Autodesk Inventor part; units mm, degrees
ref_plane "YZ Plane" through (0, 0, 0) normal (1, 0, 0) x (0, 1, 0)
ref_plane "XZ Plane" through (0, 0, 0) normal (0, 1, 0) x (-1, 0, 0)
ref_plane "XY Plane" through (0, 0, 0) normal (0, 0, 1) x (1, 0, 0)
sketch "Boceto1" plane through (0, 0, 0) normal (0, 0, 1) x (1, 0, 0)
  line L0 (0, 0) -> (-25.435, 0)
  line L1 (-25.435, 0) -> (-25.435, 10.53)
  line L2 (0, 0) -> (0, 11.4) construction
  arc A0 (9.5801, 10.53) -> (-9.5801, 10.53) centre (0, 16.38) ccw
  circle A1 centre (0, 16.38) radius 4.98
  line L3 (-25.435, 10.53) -> (-9.5801, 10.53)
  line L4 (0, 0) -> (25.435, 0)
  line L5 (25.435, 0) -> (25.435, 10.53)
  line L6 (25.435, 10.53) -> (9.5801, 10.53)
  dimension "d4" = 9.96
  dimension "d0" = 25.435
  dimension "d1" = 10.53
  dimension "d2" = 11.4
  dimension "d3" = 22.45
extrude "Extrusión1" add sketch "Boceto1" along normal blind 9.95
sketch "Boceto2" plane through (-25.435, 0, 0) normal (0, -1, 0) x (1, 0, 0)
  line L0 (25.435, 0) -> (25.435, 9.95) construction
  line L1 (36.66, 9.95) -> (14.21, 9.95)
  line L2 (25.435, 4.975) -> (41.935, 4.975) construction
  line L3 (41.935, 4.975) -> (43.685, 4.975) construction
  circle A0 centre (43.685, 4.975) radius 1.75
  circle A1 centre (7.185, 4.975) radius 1.75
  point P0 (35.0151, 9.95)
  point P1 (15.8549, 9.95)
  dimension "d7" = 16.5
  dimension "d8" = 1.75
extrude "Extrusión2" cut sketch "Boceto2" against normal up to surface (10.53 mm away)
properties part number "003" material "Steel"
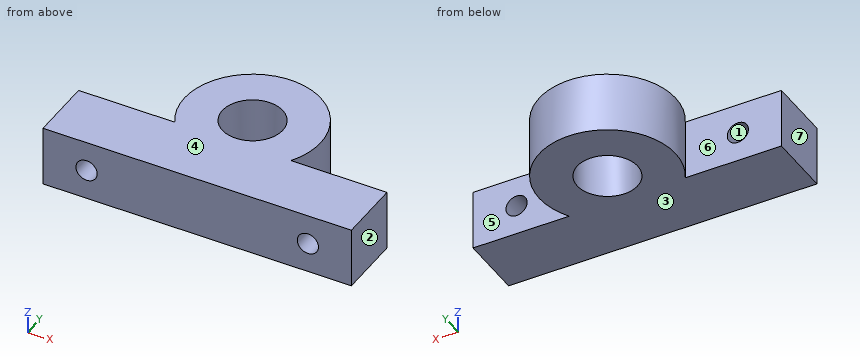
Can you work these out from the model? Positions are in its coordinate system, mm. Face numbers are marked on the shaded views. A direction names the side the tool comes from. Coordinates: 2 decimals unless noted, no trailing zeros. Loops run counter-clockwise (first coordinate to the right, second up) from the corner with the lowest first, then second, coordinate; pieces in that order, holes last. Notation, with made-up numbers: M 24,18.5 L 41,18.5 A29 cw 41,49.5 Z; hole C 40,-6 d11. An arc over 180 degrees is marked long. Return JSON: item names as keys, results as strings. Group by question number.
Item 1: On a 3-axis mill with a long thin cutter (end or side, diameter ignored), from which of +Z, -Z, +X, -X, +Y, -Y can I reach the whole of each face in a straight line? I mean the marked faces 5, 6 and 7. Say none if no direction works.
Item 2: Imagine slicing it at D-D (z = 4.25). Please give me the cut outline in (x, y) (3 decimals).
Item 3: I'm going to push flat-ended pins straight in: pin 1 Ø3 at (x, z) = (-16.5, 4.5) entering from -Y; pin 2 Ø3 at (x, z) = (-18.5, 5.5) entering from +Y. Where does each tip first touch, or does it pass through?
Item 4: Imagine slicing it at B-B (x = 0). Please give me the cut outline in (y, z) (3 decimals).
Item 5: Imagine slicing it at A-A (y = 16.38). Please give me the cut outline in (x, z) (3 decimals), and give its area (3 significant figures).
Item 6: Imagine slicing it at C-C (z = 8.75). Please give me the cut outline in (x, y) (3 decimals), and give its area (3 significant figures).
Item 7: Thinking about a two-plate mould opening in Z: for the marked faces 1, 2, 3 and 4, which applies, released by +Z, released by -Z, zero draft, split by the parting line, or undercut?
Item 8: If I drill on L1, parallel to Z at x = -18.25, y = 7.5 (3 decimals); L2, parallel to X at y = 6.75, z = 3.5 (3 decimals); L3, parallel to X at y = 2.5, z = 5.5 (3 decimals), over which ranges is the centre line in solid material (lowest first)? Write a range as from..to.
Verdict:
{
 "1": {"face 5": "+Z, -Z, +X", "face 6": "+Z, -Z, -X", "face 7": "+Z, -Z, -X, +Y, -Y"},
 "2": {"outline": "M -25.435,0 L -19.843,0 L -19.843,10.53 L -25.435,10.53 Z; M -16.657,0 L 16.657,0 L 16.657,10.53 L 9.58,10.53 A11.225 ccw long -9.58,10.53 L -16.657,10.53 Z; M 19.843,0 L 25.435,0 L 25.435,10.53 L 19.843,10.53 Z; hole C 0,16.38 d9.96"},
 "3": {"pin 1": "stops at y = 0", "pin 2": "stops at y = 10.53"},
 "4": {"outline": "M 0,0 L 11.4,0 L 11.4,9.95 L 0,9.95 Z; M 21.36,0 L 27.605,0 L 27.605,9.95 L 21.36,9.95 Z"},
 "5": {"outline": "M -11.225,0 L -4.98,0 L -4.98,9.95 L -11.225,9.95 Z; M 4.98,0 L 11.225,0 L 11.225,9.95 L 4.98,9.95 Z", "area": "124 mm^2"},
 "6": {"outline": "M -25.435,0 L 25.435,0 L 25.435,10.53 L 9.58,10.53 A11.225 ccw long -9.58,10.53 L -25.435,10.53 Z; hole C 0,16.38 d9.96", "area": "781 mm^2"},
 "7": {"face 1": "undercut", "face 2": "zero draft", "face 3": "released by -Z", "face 4": "released by +Z"},
 "8": {"L1": "z = 0..3.225, 6.725..9.95", "L2": "x = -25.435..-19.192, -17.308..17.308, 19.192..25.435", "L3": "x = -25.435..-19.919, -16.581..16.581, 19.919..25.435"}
}
